from build123d import *

# Parameters (mm, degrees)
CROQUIS1_W              = 15
CROQUIS1_H              = 15
SALIENTE_EXTRUIR1_DEPTH = 5
CROQUIS2_R              = 2.6
CORTAR_EXTRUIR1_DEPTH   = 5
CROQUIS3_W              = 12.5
CROQUIS3_H              = 12.5
CORTAR_EXTRUIR2_DEPTH   = 2


with BuildPart() as part:
    # Croquis1 → Saliente-Extruir1 (new body)
    with BuildSketch(Plane(origin=(0, 0, 0), x_dir=(1, 0, 0), z_dir=(0, 1, 0))):
        with Locations((7.5, 7.5)):
            Rectangle(CROQUIS1_W, CROQUIS1_H)
    extrude(amount=SALIENTE_EXTRUIR1_DEPTH)

    # Croquis2 → Cortar-Extruir1 (cut)
    with BuildSketch(Plane(origin=(0, 5, 0), x_dir=(1, 0, 0), z_dir=(0, 1, 0))):
        with Locations(Location((7.5, 7.5, 0), (0, 0, 270))):
            Circle(CROQUIS2_R)
    extrude(amount=-CORTAR_EXTRUIR1_DEPTH, mode=Mode.SUBTRACT)

    # Croquis3 → Cortar-Extruir2 (cut)
    with BuildSketch(Plane.XZ):
        with Locations((6.25, -8.75)):
            Rectangle(CROQUIS3_W, CROQUIS3_H)
    extrude(amount=-CORTAR_EXTRUIR2_DEPTH, mode=Mode.SUBTRACT)


solid = part.part
Input: part model. Units: mm. Frame: model coordinates. A direction names the side the tool comes from. Coordinates: 2 decimals unless noted, no trailing zeros. Loops run counter-clockwise (first coordinate to the right, second up) from the corner with the lowest first, then second, coordinate; pieces in that order, holes last. Notation, with made-up numbers: (73.5, 45) -> (130.5, 45) arc R33 ccw to (130.5, 80) -> close; hole circle Ø3 at (-15.75, 43). An arc over 180 degrees is marked (long way). Write each question's results on one line, items separated by ' | '. Start each with the question number.
Q1. Section B-B, the plane x = 7.5. Return the cut outline in (y, z).
Q2. Section A-A, the plane z = -7.5. Return the cut outline in (x, y).
Q3. Section D-D, the plane y = 0.75. Return the cut outline in (x, z).
Q4. Ray query, line 1 (X direction, y = 4.35, z = -7.5); line 2 (Z direction, x = 11.5, y = 0.85); line 3 (Y direction, x = 6.75, z = -3.5). Return the intervals inside material, ascending. Write a range as from..to.
Q5. Pull-direction query (Z, two-part tool) for faces 1 (the cylindrical face through (5.193, 3.521, -6.3)), 2 (the flat face through (6, 1, -2.5)), 3 (the flat face through (4, 5, -8)); classes: released by +Z, released by -Z, zero draft, split by the parting line, or undercut.
Q6. Pin query (flat end, axial travel): pin 1 (4 mm diameter, centred on x = 8, z = -8, fed in from -Y); pin 2 (1 mm diameter, centred on y = 1, z = -9, fed in from -X); pin 3 (0.6 mm diameter, centred on x = 8, y = 0.5, fed in from -Z); pin 4 (2 mm diameter, centred on x = 3.5, y = 3.5, fed in from +Z). Return the tip coordinate at first contact, or that it passes through.
Q7. Section C-C, the plane y = 2.8. Return the cut outline in (x, z), plus the area to 3 significant figures.
Q8. Reachability of faces 4 (the flat face through (7, 4, -15)), 5 (the flat face through (12.5, 1, -9)) from +Z, -Z, +X, -X, +Y, -Y: full face, straight path, thin tool, end or side. Return the list, or none.
Found:
1) outline: (0, -2.5) -> (2, -2.5) -> (2, -4.9) -> (5, -4.9) -> (5, 0) -> (0, 0) -> close; (2, -15) -> (5, -15) -> (5, -10.1) -> (2, -10.1) -> close
2) outline: (0, 2) -> (4.9, 2) -> (4.9, 5) -> (0, 5) -> close; (10.1, 2) -> (12.5, 2) -> (12.5, 0) -> (15, 0) -> (15, 5) -> (10.1, 5) -> close
3) outline: (0, -2.5) -> (12.5, -2.5) -> (12.5, -15) -> (15, -15) -> (15, 0) -> (0, 0) -> close
4) line 1: 0..4.9, 10.1..15 | line 2: -2.5..0 | line 3: 2..5
5) face 1: undercut | face 2: released by -Z | face 3: zero draft
6) pin 1: y = 2 | pin 2: x = 12.5 | pin 3: z = -2.5 | pin 4: z = 0
7) outline: (0, -15) -> (15, -15) -> (15, 0) -> (0, 0) -> close; hole circle Ø5.2 at (7.5, -7.5) | area: 204 mm2
8) face 4: -Z, +X, -X, +Y, -Y | face 5: -Z, -X, -Y
